Study the drawing (mm; zero at the part's minimum x, y, z) and answer. Round coordinates to 2 decimals unless told otherwise and drop trailing zeros. Order: outer loops, then holes, each group sorted by start corner. A loop starts at its lowest first (then second) coordinate and runs counter-clockwise, first axis right, second up. Notation, with made-up numbers: (1.25, 3) - (48.25, 3) arc R15 ccw to (48.25, 8) - close; hole circle Ø8 at (36.25, 72.25). An arc over 180 degrees is marked (long way). Use one line per item in the form item = value. Start each with the question number.
Q1. Given P1, Ø2, axis at x = 56, z = 11, coming from the -Y side; P2, Ø3.5, axis at y = 53, z = 10.5, coming from the -X side; P3, Ø12, axis at x = 183, z = 6.5, coming from the +Y side, each flat-ended and moving along its own axis, determine where each tip first touches the part or whether it passes through.
Q2. The part is cut by section B-B on y = 916. Determine the outline of the cut face in (x, z), plus the area to 3 significant figures.
Q3. The part is cut by section C-C on x = 448. Determine the outline of the cut face in (y, z).
Q4. Find the intervals of material crossed by line 1 (X direction, y = 46, z = 12); line 2 (Y direction, x = 653.5, z = 15.5) (1 decimal); line 3 (Y direction, x = 397, z = 10) (1 decimal), in increasing order. Write a range as [from, to].
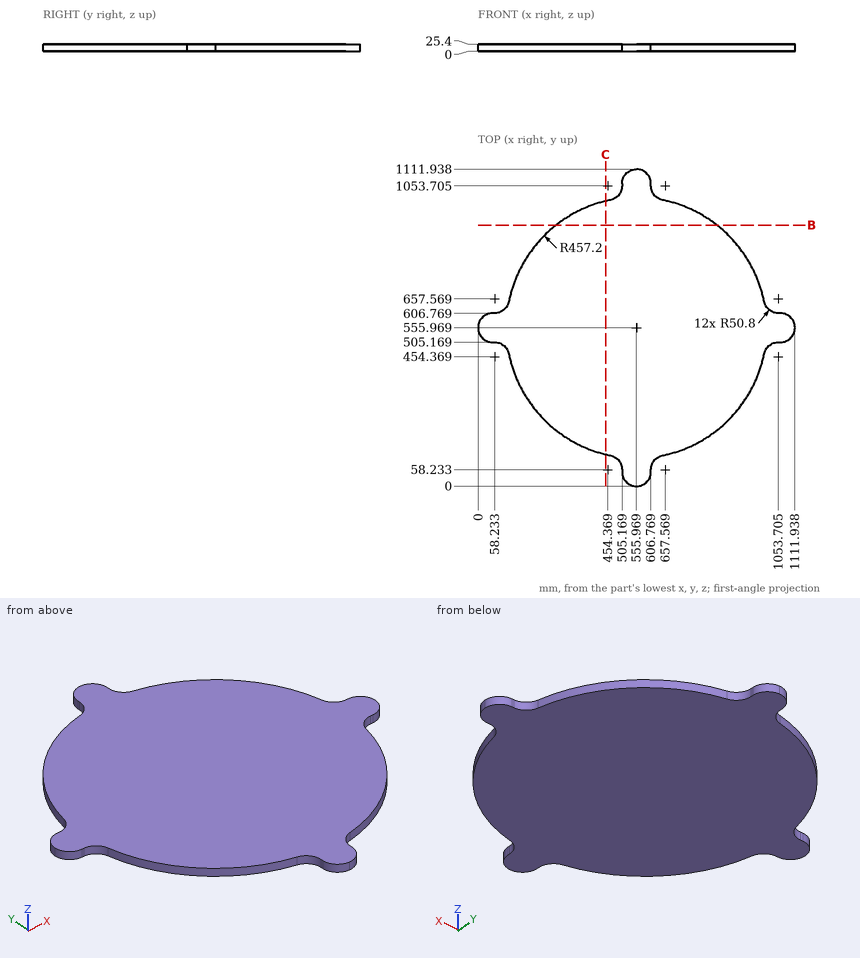
Found:
q1.P1 = 505.17
q1.P2 = 505.17
q1.P3 = 828.67
q2.outline = (274.17, 0) - (837.77, 0) - (837.77, 25.4) - (274.17, 25.4) - close
q2.area = 14,300 mm²
q3.outline = (111.7, 0) - (1000.24, 0) - (1000.24, 25.4) - (111.7, 25.4) - close
q4.line_1 = [505.4, 606.54]
q4.line_2 = [109.3, 1002.6]
q4.line_3 = [127.3, 984.6]
